Could you check a few things on this model? Use its own coordinates, in mm. A direction names the side the tool comes from. Give positions to 0.01 mm unless a question says otherwise; leave off trailing zeros. Write each question's results on one line, items separated by ' | '. Start each with the question number.
(1) On a 3-axis mill with a long thin cutter (end or side, diameter ignored), from which of +Z, -Z, +X, -X, +Y, -Y can I reach the whole of each face in a straight line? I mean faces 1 (the face through (-15.195, -38.633, -8.944)), 2 (the face through (1, -76.2, 0)). Say none if no direction works.
(2) I need wall thicknesses on line 1 (Z direction, x = 30.5, y = -44); line 2 (Z direction, x = -12, y = -63.5); line 3 (Z direction, x = 4.5, y = -9). Which ranges of each line are inside material? Lowest first, please.
(3) If we mould it in two halves opening along X, with no side actions, what happens to faces 3 (the face through (5, 0, 2)), 4 (the face through (35.796, -38.633, 4.624)), 5 (the face through (-44.475, -47.1, 10.904))? For each: released by +X, released by -X, zero draft, split by the parting line, or undercut.
(4) Suppose I cut it at A-A (y = -64.5). Count the separate pieces of the cut face and the enclosed holes in it, and give its area (3 significant figures).
(5) For pin 1 (4 mm diameter, centred on x = 1.5, y = -17, fed in from -Z); pin 2 (4 mm diameter, centred on y = -48, z = 8.5, fed in from +X); pin 3 (16.5 mm diameter, centred on x = -33.5, y = -47.5, fed in from +Z); pin 4 (1.5 mm diameter, centred on x = 40.5, z = -19, fed in from +Y), each with a flat end and sliding along its axis, tell me the tip position at first contact or that it passes through.
from build123d import *

# Parameters (mm, degrees)
F0_W     = 87.8357961774
F0_H     = 56.9998249412
F1_DEPTH = 76.2
F1_TAPER = -10
F2_R     = 15.3943409372
F3_DEPTH = 76.2010001


with BuildPart() as f1:
    # F0 (on Front) → F1 (new body)
    with BuildSketch(Plane.XZ):
        with Locations((2.1024532616, -0.116802752)):
            Rectangle(F0_W, F0_H)
    extrude(amount=F1_DEPTH, taper=F1_TAPER)

    # F2 (on face) → F3 (cut, through all)
    with BuildSketch(Plane.XZ.offset(76.2)):
        with Locations((21.1121719331, 0)):
            Circle(F2_R)
        Polygon((-40.5855899055, -17.6404323429), (-20.216173182, -17.6404323429), (-10.0314648202, 0), (-20.216173182, 17.6404323429), (-40.5855899055, 17.6404323429), (-50.7702982673, 0), align=None)
    extrude(amount=-F3_DEPTH, mode=Mode.SUBTRACT)


solid = f1.part
Output values:
1) face 1: +Y, -Y | face 2: +Z, -Z, +X, -X, -Y
2) line 1: -36.38 to -12.2, 12.2 to 36.14 | line 2: -39.81 to -3.41, 3.41 to 39.58 | line 3: -30.2 to 29.97
3) face 3: zero draft | face 4: undercut | face 5: undercut
4) separate pieces: 1 | enclosed holes: 2 | area: 7,000 mm2
5) pin 1: z = -31.97 | pin 2: x = 54.84 | pin 3: z = 38.21 | pin 4: y = 0
